from build123d import *

# Parameters (mm, degrees)
BOX009_W          = 36.4
BOX009_H          = 24.6
BOX009_DEPTH      = 6.5
BOX008_W          = 38.8
BOX008_H          = 27
BOX008_DEPTH      = 6.5
CYLINDER008_R     = 1.2
CYLINDER008_DEPTH = 10
ARRAY012_X_COUNT  = 2
ARRAY012_X_PITCH  = 29.6
ARRAY012_Y_COUNT  = 2
ARRAY012_Y_PITCH  = 17.8
BOX011_W          = 4.6
BOX011_H          = 1
BOX011_DEPTH      = 10
CYLINDER004_R     = 1.5
CYLINDER004_DEPTH = 10
CYLINDER005_R     = 2.3
CYLINDER005_DEPTH = 10
ARRAY004_X_COUNT  = 2
ARRAY004_X_PITCH  = 11.8
BOX006_W          = 36.4
BOX006_H          = 24.6
BOX006_DEPTH      = 0.5
CYLINDER_R        = 1.2
CYLINDER_DEPTH    = 10
ARRAY001_X_COUNT  = 2
ARRAY001_X_PITCH  = 29.6
ARRAY001_Y_COUNT  = 2
ARRAY001_Y_PITCH  = 17.8
BOX003_W          = 23.6
BOX003_H          = 11.8
BOX003_DEPTH      = 10
BOX007_W          = 36.4
BOX007_H          = 24.6
BOX007_DEPTH      = 0.5


with BuildPart() as outer_wall_hole_cube:
    # Box009 → Box009 (new body)
    with BuildSketch(Plane(origin=(-0.4, -0.4, 0), x_dir=(1, 0, 0), z_dir=(0, 0, 1))):
        with Locations((18.2, 12.3)):
            Rectangle(BOX009_W, BOX009_H)
    extrude(amount=BOX009_DEPTH)


with BuildPart() as outer_wall_cut:
    # Box008 → Box008 (new body)
    with BuildSketch(Plane(origin=(-1.6, -1.6, 0), x_dir=(1, 0, 0), z_dir=(0, 0, 1))):
        with Locations((19.4, 13.5)):
            Rectangle(BOX008_W, BOX008_H)
    extrude(amount=BOX008_DEPTH)

    # Cut004: cut outer wall hole cube
    add(outer_wall_hole_cube.part, mode=Mode.SUBTRACT)


with BuildPart() as outer_wall_cut_1:
    # Cut004 placement: moved
    add(outer_wall_cut.part.moved(Location((0, 0, -5.5))))


with BuildPart() as bolt_hole003:
    # Cylinder008 → Cylinder008 (new body)
    with BuildSketch(Plane.XY.offset(-10)):
        Circle(CYLINDER008_R)
    extrude(amount=CYLINDER008_DEPTH)


with BuildPart() as bolt_hole_fusion_array:
    # Cone → Cone (revolve)
    with BuildSketch(Plane.XZ):
        Polygon((0, 0), (1.2, 0), (2, 1), (0, 1), align=None)
    revolve(axis=Axis((0, 0, 0), (0, 0, 1)))

    # Fusion011: union bolt hole003
    add(bolt_hole003.part)

    # Array012 X: bolt hole fusion array ×2


with BuildPart() as bolt_hole_fusion_array_1:
    add(bolt_hole_fusion_array.part)
    with Locations(*[(i * ARRAY012_X_PITCH, 0, 0) for i in range(1, ARRAY012_X_COUNT)]):
        add(bolt_hole_fusion_array.part)

    # Array012 Y: bolt hole fusion array ×2


with BuildPart() as bolt_hole_fusion_array_2:
    add(bolt_hole_fusion_array_1.part)
    with Locations(*[(0, i * ARRAY012_Y_PITCH, 0) for i in range(1, ARRAY012_Y_COUNT)]):
        add(bolt_hole_fusion_array_1.part)


with BuildPart() as bolt_hole_fusion_array_3:
    # Array012 placement: moved
    add(bolt_hole_fusion_array_2.part.moved(Location((3, 3, 0))))


with BuildPart() as obj1:
    # Box011 → Box011 (new body)
    with BuildSketch(Plane(origin=(-2.3, -0.5, 0), x_dir=(1, 0, 0), z_dir=(0, 0, 1))):
        with Locations((2.3, 0.5)):
            Rectangle(BOX011_W, BOX011_H)
    extrude(amount=BOX011_DEPTH)


with BuildPart() as obj2:
    # Cylinder004 → Cylinder004 (new body)
    with BuildSketch(Plane.XY):
        Circle(CYLINDER004_R)
    extrude(amount=CYLINDER004_DEPTH)

    # Fusion008: union obj1
    add(obj1.part)


with BuildPart() as top_hole_fusion:
    # Cylinder005 → Cylinder005 (new body)
    with BuildSketch(Plane.XY.offset(-9.5)):
        Circle(CYLINDER005_R)
    extrude(amount=CYLINDER005_DEPTH)

    # Cut006: cut obj2
    add(obj2.part, mode=Mode.SUBTRACT)

    # Array004 X: top hole fusion ×2


with BuildPart() as top_hole_fusion_1:
    add(top_hole_fusion.part)
    with Locations(*[(i * ARRAY004_X_PITCH, 0, 0) for i in range(1, ARRAY004_X_COUNT)]):
        add(top_hole_fusion.part)


with BuildPart() as top_hole_fusion_2:
    # Array004 placement: moved
    add(top_hole_fusion_1.part.moved(Location((11.9, 11.9, 0))))

    # Fusion004: union bolt hole fusion array
    add(bolt_hole_fusion_array_3.part)


with BuildPart() as thin_top_plate:
    # Box006 → Box006 (new body)
    with BuildSketch(Plane(origin=(-0.4, -0.4, 0.5), x_dir=(1, 0, 0), z_dir=(0, 0, 1))):
        with Locations((18.2, 12.3)):
            Rectangle(BOX006_W, BOX006_H)
    extrude(amount=BOX006_DEPTH)


with BuildPart() as bolt_hole_array_clone:
    # Cylinder → Cylinder (new body)
    with BuildSketch(Plane.XY):
        Circle(CYLINDER_R)
    extrude(amount=CYLINDER_DEPTH)

    # Array001 X: bolt hole array clone ×2


with BuildPart() as bolt_hole_array_clone_1:
    add(bolt_hole_array_clone.part)
    with Locations(*[(i * ARRAY001_X_PITCH, 0, 0) for i in range(1, ARRAY001_X_COUNT)]):
        add(bolt_hole_array_clone.part)

    # Array001 Y: bolt hole array clone ×2


with BuildPart() as bolt_hole_array_clone_2:
    add(bolt_hole_array_clone_1.part)
    with Locations(*[(0, i * ARRAY001_Y_PITCH, 0) for i in range(1, ARRAY001_Y_COUNT)]):
        add(bolt_hole_array_clone_1.part)


with BuildPart() as bolt_hole_array_clone_3:
    # Array001 placement: moved
    add(bolt_hole_array_clone_2.part.moved(Location((3, 3, 0))))


with BuildPart() as mesh_extraction_fusion_clone:
    # Box003 → Box003 (new body)
    with BuildSketch(Plane(origin=(6, 6, 0), x_dir=(1, 0, 0), z_dir=(0, 0, 1))):
        with Locations((11.8, 5.9)):
            Rectangle(BOX003_W, BOX003_H)
    extrude(amount=BOX003_DEPTH)

    # Fusion003: union bolt hole array clone
    add(bolt_hole_array_clone_3.part)


with BuildPart() as top_cover_plate_fusion:
    # Box007 → Box007 (new body)
    with BuildSketch(Plane(origin=(-0.4, -0.4, 0), x_dir=(1, 0, 0), z_dir=(0, 0, 1))):
        with Locations((18.2, 12.3)):
            Rectangle(BOX007_W, BOX007_H)
    extrude(amount=BOX007_DEPTH)

    # Cut003: cut mesh extraction fusion clone
    add(mesh_extraction_fusion_clone.part, mode=Mode.SUBTRACT)

    # Fusion012: union thin top plate
    add(thin_top_plate.part)

    # Cut002: cut top hole fusion
    add(top_hole_fusion_2.part, mode=Mode.SUBTRACT)

    # Fusion005: union outer wall cut
    add(outer_wall_cut_1.part)


solid = top_cover_plate_fusion.part
For this review, take the finished solid that the model builds, in its own axes (mm). A direction names the side the tool comes from. Coordinates: 2 decimals unless noted, no trailing zeros. Loops run counter-clockwise (first coordinate to the right, second up) from the corner with the lowest first, then second, coordinate; pieces in that order, holes last. Notation, with made-up numbers: (63, 43.25) - (70, 43.25) arc R12 cw to (70, 64.25) - close; hole circle Ø9 at (10.5, 72). An arc over 180 degrees is marked (long way). Use a Markdown table: item, result. Add a question column.
Item 1: Mouldability with a two-part tool opening along X and no side actions: class faces 1 (the face through (-1.6, 12, -2)), 2 (the face through (18, 24.2, -3)), 3 (the face through (36, 12, -3)), 4 (the face through (18, 12, 1)) as pulls with the +X half, pulls with the -X half, needs draft (parallel to the pull), parting line crosses it, or undercut.
Item 2: Insertion check: pin 1 Ø12.5 at (x, y) = (16.5, 7.5) entering from -Z; pin 2 Ø9.5 at (x, y) = (22.5, 13) entering from -Z. Each pin has a flat end and moves straight along its axis. Give the tip position at first contact, or say it passes through.
Item 3: Tool access review of faces 5 (the face through (18, 25.4, -2)), 6 (the face through (18, 12, 0.5)): name each direction out of +Z, -Z, +X, -X, +Y, -Y from which nothing blocks a thin tool from reaching the whole face with its end or side.
Item 4: For line 1 (X direction, y = 0.25, z = -0.25); line 2 (X direction, y = 10.5, z = 0.25); line 3 (Y direction, x = 27, z = -0.25), list the stretches that pass through material, from the lowest coordinate up.
Item 5: We need section A-A (x = 32.6). Give the boundary of the cut face in (y, z).
Item 6: We need section B-B (z = -3.5). Give the boundary of the cut face in (x, y), and give its area (3 significant figures).
Item 7: We need section C-C (y = 0.5). Give the boundary of the cut face in (x, z), and give its area (3 significant figures).
Item 8: We need section D-D (x = 24). Give the boundary of the cut face in (y, z).
Results list:
| question | item | result |
|---|---|---|
| 1 | face 1 | pulls with the -X half |
| 1 | face 2 | undercut |
| 1 | face 3 | undercut |
| 1 | face 4 | needs draft |
| 2 | pin 1 | stops at z = 0 |
| 2 | pin 2 | stops at z = 0.5 |
| 3 | face 5 | +Z, -Z, +X, -X, +Y |
| 3 | face 6 | -Z |
| 4 | line 1 | x = -1.6 to -0.4, 36 to 37.2 |
| 4 | line 2 | x = -1.6 to 6, 29.6 to 37.2 |
| 4 | line 3 | y = -1.6 to -0.4, 24.2 to 25.4 |
| 5 | outline | (-1.6, -5.5) - (-0.4, -5.5) - (-0.4, 0) - (1.8, 0) - (1, 1) - (-1.6, 1) - close; (4.2, 0) - (19.6, 0) - (18.8, 1) - (5, 1) - close; (22, 0) - (24.2, 0) - (24.2, -5.5) - (25.4, -5.5) - (25.4, 1) - (22.8, 1) - close |
| 6 | outline | (-1.6, -1.6) - (37.2, -1.6) - (37.2, 25.4) - (-1.6, 25.4) - close; hole (-0.4, -0.4) - (36, -0.4) - (36, 24.2) - (-0.4, 24.2) - close |
| 6 | area | 152 mm^2 |
| 7 | outline | (-1.6, -5.5) - (-0.4, -5.5) - (-0.4, 0) - (36, 0) - (36, -5.5) - (37.2, -5.5) - (37.2, 1) - (-1.6, 1) - close |
| 7 | area | 52.0 mm^2 |
| 8 | outline | (-1.6, -5.5) - (-0.4, -5.5) - (-0.4, 0) - (6, 0) - (6, 0.5) - (17.8, 0.5) - (17.8, 0) - (24.2, 0) - (24.2, -5.5) - (25.4, -5.5) - (25.4, 1) - (-1.6, 1) - close |
